```python
from build123d import *
from build123d.topology import SkipClean

# Parameters (mm, degrees)
SKETCH1_R           = 1.6
BOSS_EXTRUDE1_DEPTH = 2.5
BOSS_EXTRUDE2_START = -2.5
SKETCH1_3_W         = 15
SKETCH1_3_H         = 40
SKETCH1_3_R         = 1.7
SKETCH1_3_R_2       = 1.6
BOSS_EXTRUDE2_DEPTH = 2.5
SKETCH3_R           = 3.7
SKETCH3_R_2         = 1.7
EXTRUDE_THIN2_DEPTH = 6.29
SKETCH4_W           = 15
SKETCH4_H           = 40
CUT_EXTRUDE1_DEPTH  = 2.5
CUT_EXTRUDE2_DEPTH  = 2.5
SKETCH2_R           = 1.6
BOSS_EXTRUDE3_DEPTH = 1


with BuildPart() as part:
    # Sketch1 → Boss-Extrude1 (new body)
    # profile 1 of 8: a face of its own
    with BuildSketch(Plane(origin=(0, 0, 0), x_dir=(0, 0, -1), z_dir=(1, 0, 0))):
        with BuildLine():
            Line((7.5, 21.7), (7.5, 40))
            Line((7.5, 40), (0, 40))
            Line((0, 40), (0, 0))
            Line((0, 0), (7.5, 0))
            Line((7.5, 0), (7.5, 6.4))
            ThreePointArc((7.5, 6.4), (5.9, 8), (7.5, 9.6))
            Line((7.5, 9.6), (7.5, 18.3))
            ThreePointArc((7.5, 18.3), (5.8, 20), (7.5, 21.7))
        make_face()
    # profile 2 of 8: a face of its own
    with BuildSketch(Plane(origin=(0, 0, 0), x_dir=(0, 0, -1), z_dir=(1, 0, 0))):
        with BuildLine():
            Line((15, 40), (7.5, 40))
            Line((7.5, 40), (7.5, 21.7))
            ThreePointArc((7.5, 21.7), (8.702081528, 21.202081528), (9.2, 20))
            ThreePointArc((9.2, 20), (8.702081528, 18.797918472), (7.5, 18.3))
            Line((7.5, 18.3), (7.5, 9.6))
            ThreePointArc((7.5, 9.6), (8.63137085, 9.13137085), (9.1, 8))
            ThreePointArc((9.1, 8), (8.63137085, 6.86862915), (7.5, 6.4))
            Line((7.5, 6.4), (7.5, 0))
            Line((7.5, 0), (15, 0))
            Line((15, 0), (15, 5.883419246))
            Line((15, 5.883419246), (12.2, 4.266838493))
            Line((12.2, 4.266838493), (9.4, 5.883419246))
            Line((9.4, 5.883419246), (9.4, 9.116580754))
            Line((9.4, 9.116580754), (12.2, 10.733161507))
            Line((12.2, 10.733161507), (15, 9.116580754))
            Line((15, 9.116580754), (15, 30.883419246))
            Line((15, 30.883419246), (12.2, 29.266838493))
            Line((12.2, 29.266838493), (9.4, 30.883419246))
            Line((9.4, 30.883419246), (9.4, 34.116580754))
            Line((9.4, 34.116580754), (12.2, 35.733161507))
            Line((12.2, 35.733161507), (15, 34.116580754))
            Line((15, 34.116580754), (15, 40))
        make_face()
    # profile 3 of 8: a face of its own
    with BuildSketch(Plane(origin=(0, 0, 0), x_dir=(0, 0, -1), z_dir=(1, 0, 0))):
        with BuildLine():
            ThreePointArc((9.1, 8), (8.63137085, 9.13137085), (7.5, 9.6))
            Line((7.5, 9.6), (7.5, 6.4))
            ThreePointArc((7.5, 6.4), (8.63137085, 6.86862915), (9.1, 8))
        make_face()
    # profile 4 of 8: a face of its own
    with BuildSketch(Plane(origin=(0, 0, 0), x_dir=(0, 0, -1), z_dir=(1, 0, 0))):
        with BuildLine():
            Line((7.5, 6.4), (7.5, 9.6))
            ThreePointArc((7.5, 9.6), (5.9, 8), (7.5, 6.4))
        make_face()
    # profile 5 of 8: a face of its own
    with BuildSketch(Plane(origin=(0, 0, 0), x_dir=(0, 0, -1), z_dir=(1, 0, 0))):
        with BuildLine():
            ThreePointArc((9.1, 8), (8.63137085, 9.13137085), (7.5, 9.6))
            Line((7.5, 9.6), (7.5, 6.4))
            ThreePointArc((7.5, 6.4), (8.63137085, 6.86862915), (9.1, 8))
        make_face()
    # profile 6 of 8: a face of its own
    with BuildSketch(Plane(origin=(0, 0, 0), x_dir=(0, 0, -1), z_dir=(1, 0, 0))):
        with BuildLine():
            Line((7.5, 6.4), (7.5, 9.6))
            ThreePointArc((7.5, 9.6), (5.9, 8), (7.5, 6.4))
        make_face()
    # profile 7 of 8: a face of its own
    with BuildSketch(Plane(origin=(0, 0, 0), x_dir=(0, 0, -1), z_dir=(1, 0, 0))):
        Polygon((15, 5.883419246), (15, 9.116580754), (12.2, 10.733161507), (9.4, 9.116580754), (9.4, 5.883419246), (12.2, 4.266838493), align=None)
        with Locations((12.2, 7.5)):
            Circle(SKETCH1_R, mode=Mode.SUBTRACT)
    # profile 8 of 8: a face of its own
    with BuildSketch(Plane(origin=(0, 0, 0), x_dir=(0, 0, -1), z_dir=(1, 0, 0))):
        Polygon((15, 30.883419246), (15, 34.116580754), (12.2, 35.733161507), (9.4, 34.116580754), (9.4, 30.883419246), (12.2, 29.266838493), align=None)
        with Locations((12.2, 32.5)):
            Circle(SKETCH1_R, mode=Mode.SUBTRACT)
    extrude(amount=BOSS_EXTRUDE1_DEPTH)

    # Sketch1<3> → Boss-Extrude2 (add)
    with SkipClean():  # the faces are left unmerged after this step: merging them gives an invalid solid
        with BuildSketch(Plane(origin=(0, 0, 0), x_dir=(0, 0, -1), z_dir=(1, 0, 0)).offset(BOSS_EXTRUDE2_START)):
            with Locations((7.5, 20)):
                Rectangle(SKETCH1_3_W, SKETCH1_3_H)
            with Locations((7.5, 20)):
                Circle(SKETCH1_3_R, mode=Mode.SUBTRACT)
            with Locations((12.2, 32.5)):
                Circle(SKETCH1_3_R_2, mode=Mode.SUBTRACT)
            with Locations((12.2, 7.5)):
                Circle(SKETCH1_3_R_2, mode=Mode.SUBTRACT)
        extrude(amount=BOSS_EXTRUDE2_DEPTH)


with BuildPart() as part_1:
    # Body-Move/Copy1: moved
    add(part.part.moved(Location((-5, 0, 0))))

    # Sketch3 → Extrude-Thin2 (add)
    with SkipClean():  # the faces are left unmerged after this step: merging them gives an invalid solid
        with BuildSketch(Plane(origin=(-2.5, 0, 0), x_dir=(0, 0, -1), z_dir=(1, 0, 0))):
            with Locations((7.5, 20)):
                Circle(SKETCH3_R)
            with Locations((7.5, 20)):
                Circle(SKETCH3_R_2, mode=Mode.SUBTRACT)
        extrude(amount=EXTRUDE_THIN2_DEPTH)
    add(part_1.part.scale(1), mode=Mode.REPLACE)  # the faces are merged on a copy

    # Sketch4 → Cut-Extrude1 (cut)
    with BuildSketch(Plane.ZY.offset(7.5)):
        with Locations((-7.5, 20)):
            Rectangle(SKETCH4_W, SKETCH4_H)
    extrude(amount=-CUT_EXTRUDE1_DEPTH, mode=Mode.SUBTRACT)

    # Sketch5 → Cut-Extrude2 (cut)
    with BuildSketch(Plane.ZY.offset(5)):
        with BuildLine():
            ThreePointArc((0, 33.564659966), (-2.979157617, 27.071067812), (-4, 20))
            Line((-4, 20), (0, 20))
            Line((0, 20), (0, 33.564659966))
        make_face()
        with BuildLine():
            Line((0, 20), (-4, 20))
            ThreePointArc((-4, 20), (-2.979157617, 12.928932188), (0, 6.435340034))
            Line((0, 6.435340034), (0, 20))
        make_face()
        with BuildLine():
            Line((0, 33.564659966), (0, 20))
            Line((0, 20), (0, 6.435340034))
            ThreePointArc((0, 6.435340034), (28.071067812, -3.979157617), (46, 20))
            ThreePointArc((46, 20), (28.071067812, 43.979157617), (0, 33.564659966))
        make_face()
    extrude(amount=-CUT_EXTRUDE2_DEPTH, mode=Mode.SUBTRACT)

    # Sketch2 → Boss-Extrude3 (add)
    # profile 1 of 2: a face of its own
    with BuildSketch(Plane.ZY.offset(2.5)):
        with BuildLine():
            Line((-15, 9.7627417), (-15, 5.2372583))
            ThreePointArc((-15, 5.2372583), (-11, 4.10588745), (-8.6, 7.5))
            ThreePointArc((-8.6, 7.5), (-11, 10.89411255), (-15, 9.7627417))
        make_face()
        with Locations((-12.2, 7.5)):
            Circle(SKETCH2_R, mode=Mode.SUBTRACT)
    # profile 2 of 2: a face of its own
    with BuildSketch(Plane.ZY.offset(2.5)):
        with BuildLine():
            Line((-15, 34.7627417), (-15, 30.2372583))
            ThreePointArc((-15, 30.2372583), (-11, 29.10588745), (-8.6, 32.5))
            ThreePointArc((-8.6, 32.5), (-11, 35.89411255), (-15, 34.7627417))
        make_face()
        with Locations((-12.2, 32.5)):
            Circle(SKETCH2_R, mode=Mode.SUBTRACT)
    extrude(amount=-BOSS_EXTRUDE3_DEPTH)


solid = part_1.part
```
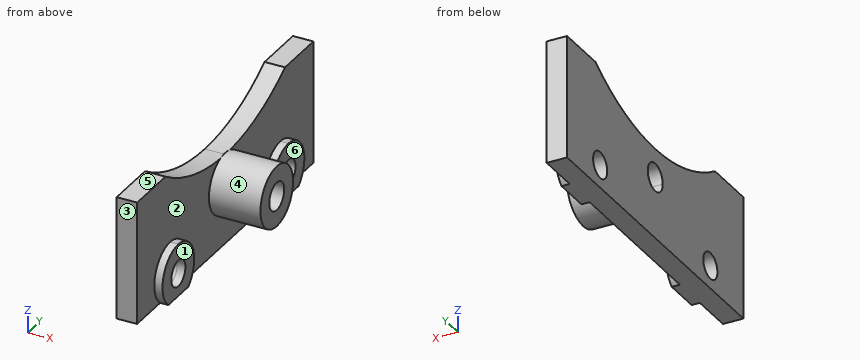
Design review of the part built by this model. Coordinates are the model's own, in mm. Face numbers are marked on the shaded views. A direction names the side the tool comes from. Round coordinates to 2 decimals unless told otherwise and drop trailing zeros. Write each loop counter-clockwise with the first axis right and the second up, starting at its lowest first coordinate (ties: lowest second). Pieces come first, ordered by that corner, then holes. Notation, with made-up numbers: (86.25, -1.75) -> (111.25, -1.75) arc R32 ccw to (111.25, 31.25) -> close; hole circle Ø1 at (-24, -31). An arc over 180 degrees is marked (long way). Write item = value, one per line. Start each with the question number.
1) Wall thickness on probe 1 along Y at (x, z) = (-3.45, -12.2); probe 2 along Z at (x, y) = (2.5, 20); probe 3 along Y at (x, z) = (-2.2, -12.2): over which ranges is each line inside the solid? List them lowest first. Write a range as from..to.
2) Take a section at D-D, the plane y = 25. State the section outline as (x, z) points.
3) Tool access review of the marked faces 4, 5 and 6: name each direction out of +Z, -Z, +X, -X, +Y, -Y from which nothing blocks a thin tool from reaching the whole face with its end or side.
4) Take a section at C-C, the plane z = -4.5. State the section outline as (x, y) points, plus the area to 3 significant figures.
5) Take a section at A-A, the plane z = -1.25. State the section outline as (x, y) points.
6) Clearance check with flat-ended pins moving along their axes: pin 1 (5 mm diameter, centred on y = 10.5, z = -3, fed in from +X); pin 2 (3 mm diameter, centred on y = 7.5, z = -12.2, fed in from +X); pin 3 (3 mm diameter, centred on x = 1.5, y = 18.5, fed in from +Z); pin 4 (4 mm diameter, centred on y = 20, z = -7.5, fed in from -X). State where each tip first meets the part, or that it passes through.
7) Mouldability with a two-part tool opening along Y and no side actions: class the marked faces 1, 2 and 3 as +Y half, -Y half, draft (parallel to the pull), parting line (faces both ways), or undercut.
8) Take a section at B-B, the plane x = 3.25. State the section outline as (y, z) points.
Results list:
q1.probe_1 = 0..5.9, 9.1..30.9, 34.1..40
q1.probe_2 = -11.2..-9.2, -5.8..-3.8
q1.probe_3 = 3.9..5.9, 9.1..11.1, 28.9..30.9, 34.1..36.1
q2.outline = (-5, -15) -> (-2.5, -15) -> (-2.5, -3.49) -> (-5, -3.49) -> close
q3.face_4 = +X
q3.face_5 = +Z, +X, -X, +Y, -Y
q3.face_6 = +Z, -Z, +X, +Y
q4.outline = (-5, 0) -> (-2.5, 0) -> (-2.5, 17.83) -> (3.79, 17.83) -> (3.79, 22.17) -> (-2.5, 22.17) -> (-2.5, 40) -> (-5, 40) -> close
q4.area = 127 mm²
q5.outline = (-5, 0) -> (-2.5, 0) -> (-2.5, 8.6) -> (-5, 8.6) -> close; (-5, 31.4) -> (-2.5, 31.4) -> (-2.5, 40) -> (-5, 40) -> close
q6.pin_1 = -2.5
q6.pin_2 = through
q6.pin_3 = -3.8
q6.pin_4 = -5
q7.face_1 = draft
q7.face_2 = undercut
q7.face_3 = -Y half
q8.outline = circle Ø7.4 at (20, -7.5); hole circle Ø3.4 at (20, -7.5)
